```python
from build123d import *

# Parameters (mm, degrees)
BOSS_EXTRUDE2_DEPTH = 11.5
CUT_EXTRUDE1_REACH  = 46.232
SKETCH4_R           = 1.5
CUT_EXTRUDE2_REACH  = 39.699
FILLET2_R           = 1


with BuildPart() as part:
    # Sketch3 → Boss-Extrude2 (new body)
    with BuildSketch(Plane(origin=(0, 0, 0), x_dir=(1, 0, 0), z_dir=(0, 1, 0))):
        Polygon((-19.5, 3), (-11.5, 3), (-11.5, 0), (-17.4, 0), (-17.4, -35), (-19.5, -35), align=None)
    extrude(amount=BOSS_EXTRUDE2_DEPTH)

    # Sketch4 → Cut-Extrude1 (cut, up to next)
    with BuildSketch(Plane(origin=(0, 0, -3), x_dir=(-1, 0, 0), z_dir=(0, 0, -1)), mode=Mode.PRIVATE) as cut_extrude1_sk1:
        with Locations((13.9, 5.75)):
            Circle(SKETCH4_R)
    cut_extrude1_tool1 = extrude(cut_extrude1_sk1.sketch, amount=-CUT_EXTRUDE1_REACH, mode=Mode.PRIVATE) & part.part
    add(cut_extrude1_tool1.solids().sort_by_distance((-13.9, 5.75, -3))[0], mode=Mode.SUBTRACT)

    # Sketch5 → Cut-Extrude2 (cut, up to next)
    with BuildSketch(Plane.ZY.offset(19.5), mode=Mode.PRIVATE) as cut_extrude2_sk1:
        with BuildLine():
            Line((27, 3.947224362), (27, 7.552775638))
            ThreePointArc((27, 7.552775638), (33.5, 5.75), (27, 3.947224362))
        make_face()
    cut_extrude2_tool1 = extrude(cut_extrude2_sk1.sketch, amount=-CUT_EXTRUDE2_REACH, mode=Mode.PRIVATE) & part.part
    add(cut_extrude2_tool1.solids().sort_by_distance((-19.5, 5.75, 30.104819))[0], mode=Mode.SUBTRACT)

    # Fillet2
    # the kernel refuses this fillet: 1 mm, written as the material it adds along each edge
    with BuildSketch(Plane(origin=(-17.4, 0, 0), x_dir=(1, 0, 0), z_dir=(0, 1, 0))) as fillet2_piece_1:
        with BuildLine():
            CenterArc((FILLET2_R, -FILLET2_R), FILLET2_R, 90, 90)
            Line((0, -FILLET2_R), (0, 0))
            Line((0, 0), (FILLET2_R, 0))
        make_face()
    extrude(amount=11.5)
    # the kernel refuses this fillet: 1 mm, written as the material it takes off along each edge
    with BuildSketch(Plane(origin=(-19.5, -2.5, -3), x_dir=(1, 0, 0), z_dir=(0, 1, 0))) as fillet2_2_piece_1:
        with BuildLine():
            CenterArc((FILLET2_R, -FILLET2_R), FILLET2_R, 90, 90)
            Line((0, -FILLET2_R), (0, 0))
            Line((0, 0), (FILLET2_R, 0))
        make_face()
    extrude(amount=16.5, mode=Mode.SUBTRACT)
    with BuildSketch(Plane(origin=(-11.5, -2.5, -3), x_dir=(-1, 0, 0), z_dir=(0, 1, 0)), Plane(origin=(-11.5, -2.5, 0), x_dir=(0, 0, -1), z_dir=(0, 1, 0))) as fillet2_2_piece_2:
        with BuildLine():
            CenterArc((FILLET2_R, FILLET2_R), FILLET2_R, 180, 90)
            Line((0, FILLET2_R), (0, 0))
            Line((0, 0), (FILLET2_R, 0))
        make_face()
    extrude(amount=16.5, mode=Mode.SUBTRACT)
    with BuildSketch(Plane(origin=(-22, 11.5, -3), x_dir=(0, -1, 0), z_dir=(1, 0, 0))) as fillet2_2_piece_3:
        with BuildLine():
            CenterArc((FILLET2_R, -FILLET2_R), FILLET2_R, 90, 90)
            Line((0, -FILLET2_R), (0, 0))
            Line((0, 0), (FILLET2_R, 0))
        make_face()
    extrude(amount=13, mode=Mode.SUBTRACT)
    with BuildSketch(Plane(origin=(-22, 0, -3), x_dir=(0, 1, 0), z_dir=(1, 0, 0))) as fillet2_2_piece_4:
        with BuildLine():
            CenterArc((FILLET2_R, FILLET2_R), FILLET2_R, 180, 90)
            Line((0, FILLET2_R), (0, 0))
            Line((0, 0), (FILLET2_R, 0))
        make_face()
    extrude(amount=13, mode=Mode.SUBTRACT)


solid = part.part
```
Geometry check sheet. Reference: the model listing, model coordinates, mm. A direction names the side the tool comes from. Round coordinates to 2 decimals unless told otherwise and drop trailing zeros. Loops run counter-clockwise (first coordinate to the right, second up) from the corner with the lowest first, then second, coordinate; pieces in that order, holes last. Notation, with made-up numbers: (15.5, 38.25) - (62.5, 38.25) arc R22 cw to (62.5, 73.25) - close; hole circle Ø1 at (52, 55). An arc over 180 degrees is marked (long way). Use a Markdown table: item, result.
Q1. Material ranges on line 1 (Y direction, x = -18.25, z = 30); line 2 (Y direction, x = -13.9, z = -2.05); line 3 (X direction, y = 5.75, z = -1.65), recorded low to high.
Solutions:
| item | result |
|---|---|
| line 1 | y = 0 to 2.25, 9.25 to 11.5 |
| line 2 | y = 0 to 4.25, 7.25 to 11.5 |
| line 3 | x = -19.5 to -15.4, -12.4 to -11.5 |
Q2. Cross-section at A-A on z = 30. Record the cut outline in (x, y), plus the area to 3 significant figures.
Solutions:
| item | result |
|---|---|
| outline | (-19.5, 0) - (-17.4, 0) - (-17.4, 2.25) - (-19.5, 2.25) - close; (-19.5, 9.25) - (-17.4, 9.25) - (-17.4, 11.5) - (-19.5, 11.5) - close |
| area | 9.45 mm2 |
Q3. Go/stop test with flat-tipped pins: P1, Ø2, axis at x = -14, y = 8, coming from the +Z side; P2, Ø6, axis at y = 3, z = 13, coming from the +X side. Record where each tip stops, or that it passes through.
Solutions:
| item | result |
|---|---|
| P1 | stops at z = 0 |
| P2 | stops at x = -17.4 |
Q4. Access from +Z, -Z, +X, -X, +Y, -Y to the whole of each face (thin tool, end or side, straight path). Record for faces 1 (the flat face through (-18, 6, 27)), 2 (the flat face through (-16, 6, 0)), 3 (the cylindrical face through (-15.556, 11.199, -2.715)).
Solutions:
| item | result |
|---|---|
| face 1 | +X, -X |
| face 2 | +Z, +X, +Y, -Y |
| face 3 | -Z, +X, -X, +Y |
Q5. Cross-section at C-C on y = 3.5. Record the cut outline in (x, z).
Solutions:
| item | result |
|---|---|
| outline | (-19.5, -2) arc R1 ccw to (-18.5, -3) - (-12.5, -3) arc R1 ccw to (-11.5, -2) - (-11.5, -1) arc R1 ccw to (-12.5, 0) - (-16.4, 0) arc R1 cw to (-17.4, 1) - (-17.4, 27.32) - (-19.5, 27.32) - close; (-19.5, 32.68) - (-17.4, 32.68) - (-17.4, 35) - (-19.5, 35) - close |
Q6. Cross-section at D-D on x = -15.75. Record the cut outline in (y, z), plus the area to 3 significant figures.
Solutions:
| item | result |
|---|---|
| outline | (0, -2) arc R1 ccw to (1, -3) - (10.5, -3) arc R1 ccw to (11.5, -2) - (11.5, 0) - (0, 0) - close |
| area | 34.1 mm2 |
Q7. Cross-section at B-B on x = -13.9. Record the cut outline in (y, z), plus the area to 3 significant figures.
Solutions:
| item | result |
|---|---|
| outline | (0, -2) arc R1 ccw to (1, -3) - (4.25, -3) - (4.25, 0) - (0, 0) - close; (7.25, -3) - (10.5, -3) arc R1 ccw to (11.5, -2) - (11.5, 0) - (7.25, 0) - close |
| area | 25.1 mm2 |
Q8. Draft check along Y on faces 4 (the flat face through (-18, 0, 14)), 5 (the cylindrical face through (-12.4, 5.8, -1.5)), 6 (the flat face through (-18, 11.5, 14)). Enter one of: released by +Y, released by -Y, zero draft, split by the parting line, or undercut.
Solutions:
| item | result |
|---|---|
| face 4 | released by -Y |
| face 5 | undercut |
| face 6 | released by +Y |
